Here's how the part is built. I have some questions about the finished solid (model axes, mm). Face numbers are marked on the shaded views. A direction names the side the tool comes from. Round coordinates to 2 decimals unless told otherwise and drop trailing zeros. Loops run counter-clockwise (first coordinate to the right, second up) from the corner with the lowest first, then second, coordinate; pieces in that order, holes last. Notation, with made-up numbers: M -30,-37.5 L 13,-37.5 A29 cw 13,-15.5 Z; hole C 27,37 d10. An arc over 180 degrees is marked long. Use a Markdown table: item, result.
from build123d import *

# Parameters (mm, degrees)
BOSS_EXTRUDE1_DEPTH     = 45
CUT_EXTRUDE1_START      = -158.56066
SKETCH2_R               = 1.5
CUT_EXTRUDE1_DEPTH      = 10
CUT_EXTRUDE2_DEPTH      = 10
CUT_EXTRUDE2_DEPTH_BACK = 10
SKETCH3_R               = 1.5
CHAMFER1_SIZE           = 0.7


with BuildPart() as part:
    # Sketch1 → Boss-Extrude1 (new body)
    with BuildSketch(Plane.XY):
        with BuildLine():
            Line((2.5, -163.560660172), (12.5, -163.560660172))
            Line((12.5, -163.560660172), (12.5, -158.560660172))
            Line((12.5, -158.560660172), (3.560660172, -158.560660172))
            ThreePointArc((3.560660172, -158.560660172), (2.810660172, -158.25), (2.5, -157.5))
            Line((2.5, -157.5), (2.5, 152.5))
            Line((2.5, 152.5), (-2.5, 152.5))
            Line((-2.5, 152.5), (-2.5, -158.560660172))
            ThreePointArc((-2.5, -158.560660172), (-1.035533906, -162.096194078), (2.5, -163.560660172))
        make_face()
    extrude(amount=BOSS_EXTRUDE1_DEPTH)

    # Sketch2 → Cut-Extrude1 (cut)
    with BuildSketch(Plane(origin=(0, 0, 0), x_dir=(1, 0, 0), z_dir=(0, 1, 0)).offset(CUT_EXTRUDE1_START)):
        with Locations(Location((7.5, -15, 0), (0, 0, 270))):
            Circle(SKETCH2_R)
        with Locations(Location((7.5, -30, 0), (0, 0, 270))):
            Circle(SKETCH2_R)
    extrude(amount=-CUT_EXTRUDE1_DEPTH, mode=Mode.SUBTRACT)

    # Sketch3 → Cut-Extrude2 (cut, two sides: drawn at the far end of the back side and taken through both)
    with BuildSketch(Plane(origin=(0, 0, 0), x_dir=(0, 0, -1), z_dir=(1, 0, 0)).offset(-CUT_EXTRUDE2_DEPTH_BACK)):
        with Locations(Location((-15, 145.5, 0), (0, 0, 180))):
            Circle(SKETCH3_R)
        with Locations(Location((-30, 145.5, 0), (0, 0, 180))):
            Circle(SKETCH3_R)
    extrude(amount=CUT_EXTRUDE2_DEPTH + CUT_EXTRUDE2_DEPTH_BACK, mode=Mode.SUBTRACT)

    # Chamfer1
    chamfer1_edges = [part.edges().sort_by_distance(p)[0] for p in [
        (12.5, -158.560660172, 22.5),
    ]]
    chamfer(chamfer1_edges, length=CHAMFER1_SIZE)


solid = part.part
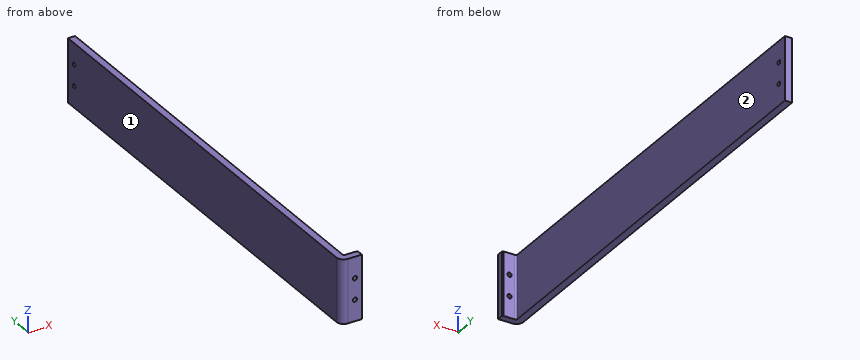
1. Which directions (+Z, -Z, +X, -X, +Y, -Y) give clear straight access to the entire face, cutting with the end or side of a thin tool? Please do the marked faces 1 and 2.
Answer sheet:
| item | result |
|---|---|
| face 1 | +Z, -Z, -X, +Y, -Y |
| face 2 | +Z, -Z, +X, +Y |
2. Imagine slicing it at A-A, the plane z = 41. Write out the boundary of the cut face in (x, y), then the cut area to 3 significant figures.
Answer sheet:
| item | result |
|---|---|
| outline | M -2.5,-158.56 A5 ccw 2.5,-163.56 L 12.5,-163.56 L 12.5,-159.26 L 11.8,-158.56 L 3.56,-158.56 A1.06 cw 2.5,-157.5 L 2.5,152.5 L -2.5,152.5 Z |
| area | 1,620 mm2 |
3. I need wall thicknesses on probe 1 along X at (y, z) = (-116.5, 30.5); probe 2 along X at (y, z) = (-161.7, 30); probe 3 along Y at (x, z) = (6.25, 42.5). Which ranges of each line are inside material? Lowest first, please. Write a range as from..to.
Answer sheet:
| item | result |
|---|---|
| probe 1 | -2.5..2.5 |
| probe 2 | -1.39..6, 9..12.5 |
| probe 3 | -163.56..-158.56 |
4. For pin 1 Ø6.5 at (x, z) = (6.5, 15.5) entering from +Y; pin 2 Ø5 at (x, z) = (7.5, 15) entering from +Y; pin 3 Ø1 at (y, z) = (4, 21) entering from +X, each with a flat end and sliding along its axis, tell me the tip position at first contact or that it passes through.
Answer sheet:
| item | result |
|---|---|
| pin 1 | y = -158.51 |
| pin 2 | y = -158.56 |
| pin 3 | x = 2.5 |
5. Imagine slicing it at B-B, the plane y = -16. Write out the boundary of the cut face in (x, z).
Answer sheet:
| item | result |
|---|---|
| outline | M -2.5,0 L 2.5,0 L 2.5,45 L -2.5,45 Z |
